from build123d import *

# Parameters (mm, degrees)
FILLET_ROUND_R          = 0.8
CHAMF_PLASTIC_BASE_SIZE = 1
SKETCH3_OUTSIDE_W       = 23.904
SKETCH3_OUTSIDE_H       = 23.904
CUT_8MM_HEX_DEPTH       = 3
SKETCH4_OUTSIDE_W       = 23.904
SKETCH4_OUTSIDE_H       = 23.904
CUT_5MM_HEX_DEPTH       = 2
BOSS_PIVOT_DEPTH        = 4
FILLET_PIVOT_R          = 0.8
CUT_EXTRUDE1_DEPTH      = 36.749562971
CUT_EXTRUDE1_DEPTH_BACK = 36.749562971
SKETCH6_W               = 4
SKETCH6_H               = 6.8
SKETCH7_R               = 1.3
CUT_EXTRUDE2_DEPTH      = 5


with BuildPart() as part:
    # Sketch1 → revolve body (revolve)
    with BuildSketch(Plane.XY, mode=Mode.PRIVATE) as revolve_body_sk:
        Polygon((6.5, 0), (6.5, 8.375), (6, 9), (6.625, 9.5), (6.625, 24), (0, 24), (0, 0), align=None)
    revolve(revolve_body_sk.sketch.rotate(Axis((0, 0, 0), (0, 1, 0)), 90), axis=Axis((0, 0, 0), (0, 1, 0)))

    # fillet round
    fillet_round_edges = [part.edges().sort_by_distance(p)[0] for p in [
        (0, 9.5, 6.625),
        (0, 24, 6.625),
    ]]
    fillet(fillet_round_edges, radius=FILLET_ROUND_R)

    # chamf plastic base
    chamf_plastic_base_edges = [part.edges().sort_by_distance(p)[0] for p in [
        (0, 0, 6.5),
    ]]
    chamfer(chamf_plastic_base_edges, length=CHAMF_PLASTIC_BASE_SIZE)

    # Sketch2 → revolve threaded body (revolve)
    with BuildSketch(Plane.XY, mode=Mode.PRIVATE) as revolve_threaded_body_sk:
        Polygon((3.2, 0), (3.2, -6), (4.5, -6), (4.5, -8), (3.25, -8), (3.25, -10), (1.3, -10), (1.3, -15), (0, -15), (0, 0), align=None)
    revolve(revolve_threaded_body_sk.sketch.rotate(Axis((0, 0, 0), (0, -1, 0)), 90), axis=Axis((0, 0, 0), (0, -1, 0)))

    # Sketch3 outside → cut 8mm hex (cut)
    with BuildSketch(Plane.XZ.offset(8)):
        Rectangle(SKETCH3_OUTSIDE_W, SKETCH3_OUTSIDE_H)
        Polygon((0, 4.618802154), (-4, 2.309401077), (-4, -2.309401077), (0, -4.618802154), (4, -2.309401077), (4, 2.309401077), align=None, mode=Mode.SUBTRACT)
    extrude(amount=-CUT_8MM_HEX_DEPTH, mode=Mode.SUBTRACT)

    # Sketch4 outside → cut 5mm hex (cut)
    with BuildSketch(Plane.XZ.offset(10)):
        Rectangle(SKETCH4_OUTSIDE_W, SKETCH4_OUTSIDE_H)
        Polygon((0, 2.886751346), (-2.5, 1.443375673), (-2.5, -1.443375673), (0, -2.886751346), (2.5, -1.443375673), (2.5, 1.443375673), align=None, mode=Mode.SUBTRACT)
    extrude(amount=-CUT_5MM_HEX_DEPTH, mode=Mode.SUBTRACT)

    # Sketch5 → boss pivot (add, symmetric)
    with BuildSketch(Plane.XY):
        with BuildLine():
            Line((-4, 24), (4, 24))
            Line((4, 24), (4, 30.5))
            ThreePointArc((4, 30.5), (0, 34.5), (-4, 30.5))
            Line((-4, 30.5), (-4, 24))
        make_face()
    extrude(amount=BOSS_PIVOT_DEPTH, both=True)

    # fillet pivot
    fillet_pivot_edges = [part.edges().sort_by_distance(p)[0] for p in [
        (-4, 27.25, -4),
        (4, 27.25, -4),
        (0, 34.5, -4),
        (-4, 27.25, 4),
        (4, 27.25, 4),
        (0, 34.5, 4),
    ]]
    fillet(fillet_pivot_edges, radius=FILLET_PIVOT_R)

    # Sketch6 → Cut-Extrude1 (cut, two sides: drawn at the far end of the back side and taken through both)
    with BuildSketch(Plane(origin=(0, 0, 0), x_dir=(0, 0, -1), z_dir=(1, 0, 0)).offset(-CUT_EXTRUDE1_DEPTH_BACK)):
        with Locations((0, 31.1)):
            Rectangle(SKETCH6_W, SKETCH6_H)
    extrude(amount=CUT_EXTRUDE1_DEPTH + CUT_EXTRUDE1_DEPTH_BACK, mode=Mode.SUBTRACT)

    # Sketch7 → Cut-Extrude2 (cut)
    with BuildSketch(Plane.XZ.offset(15)):
        Circle(SKETCH7_R)
    extrude(amount=-CUT_EXTRUDE2_DEPTH, mode=Mode.SUBTRACT)


solid = part.part
Here's how the part is built. I have some questions about the finished solid (model axes, mm). A direction names the side the tool comes from. Round coordinates to 2 decimals unless told otherwise and drop trailing zeros. Write each loop counter-clockwise with the first axis right and the second up, starting at its lowest first coordinate (ties: lowest second). Pieces come first, ordered by that corner, then holes.
1. Suppose I cut it at B-B (y = 7). List the corners of the cut face in (x, z) for me.
2. If we mould it in two halves opening along Z, with no side actions, what happens to faces 1 (the flat face through (0, 31, -2)), 2 (the flat face through (-4, 27, 0)), 3 (the flat face through (-1.267, -9.014, -2.155)), 4 (the cylindrical face through (-0.961, -3.042, 3.052))? For each: released by +Z, released by -Z, zero draft, split by the parting line, or undercut.
3. I need wall thicknesses on L1, parallel to Y at x = 4.5, z = -1.25; L2, parallel to Z at x = 1, y = 27.5; L3, parallel to Z at x = 1.75, y = 28.5. Which ranges of each line are inside material? Lowest first, please.
4. For faces 5 (the flat face through (1.233, -9.014, -2.175)), 6 (the cylindrical face through (-3.77, 27.2, -3.76)), 7 (the flat face through (2.5, -9, 0)), 8 (the flat face through (1.267, -9.014, 2.155)), which set-ups out of +Z, -Z, +X, -X, +Y, -Y let a thin tool reach every point of the face, with its end or its side?
5. Will these pins go through, and if not, where does the flat tip stop? pin 1 Ø3 at (y, z) = (27.5, 1) entering from -X; pin 2 Ø5.5 at (x, y) = (-1.5, 32) entering from +Z; pin 3 Ø5 at (x, y) = (0.5, -2) entering from -Z.
6. Suppose I cut it at A-A (y = 25.5). List the corners of the cut face in (x, z) for me.
7. Suppose I cut it at C-C (y = 0.5). List the corners of the cut face in (x, z) for me, and give its area (3 significant figures).
Answer sheet:
1. outline: circle Ø13 at (0, 0)
2. face 1: undercut
2. face 2: zero draft
2. face 3: released by -Z
2. face 4: split by the parting line
3. L1: y = 0 to 24
3. L2: z = -4 to 4
3. L3: z = -4 to -2, 2 to 4
4. face 5: -Z, +X, -Y
4. face 6: -Z, -X, +Y
4. face 7: +Z, -Z, +X, -Y
4. face 8: +Z, +X, -Y
5. pin 1: stops at x = -4
5. pin 2: stops at z = 4
5. pin 3: stops at z = -5.99
6. outline: (-4, -3.2) arc R0.8 ccw to (-3.2, -4) - (3.2, -4) arc R0.8 ccw to (4, -3.2) - (4, 3.2) arc R0.8 ccw to (3.2, 4) - (-3.2, 4) arc R0.8 ccw to (-4, 3.2) - close
7. outline: circle Ø12 at (0, 0)
7. area: 113 mm2
